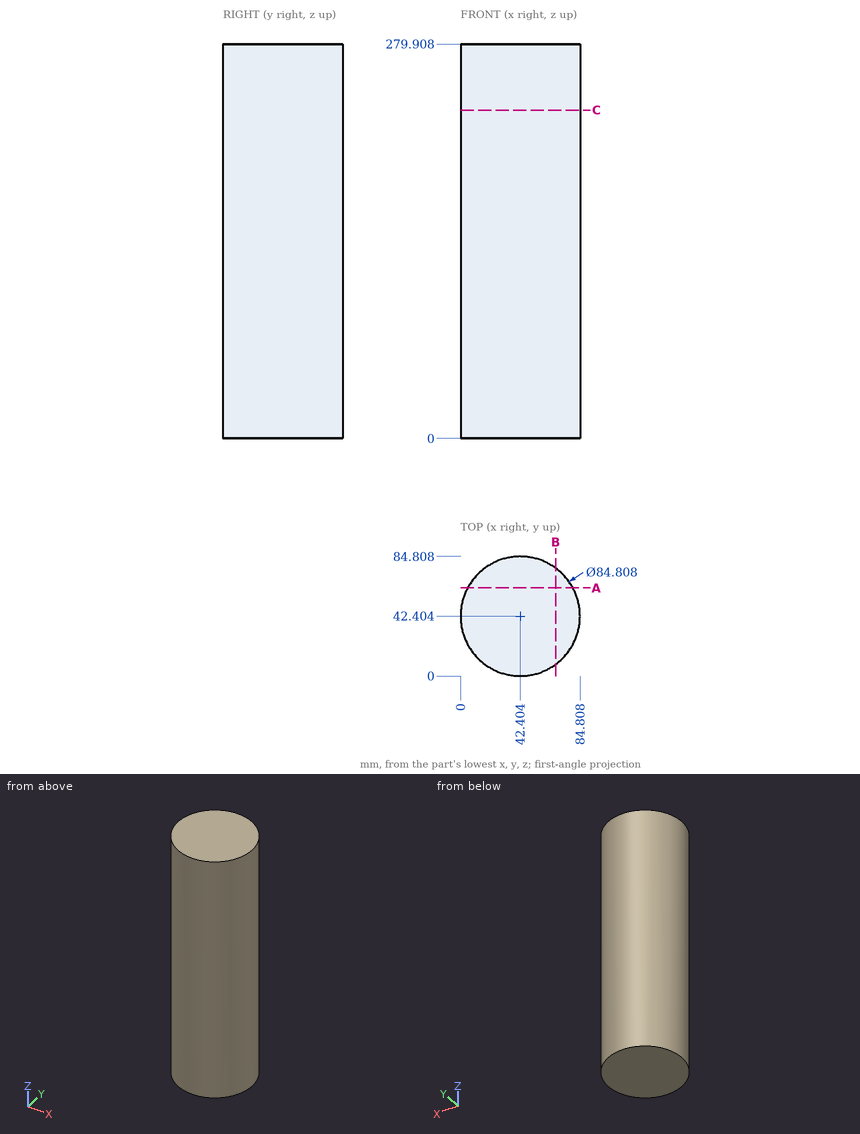
Can you work these out from the drawing? Everything is in mm from the part's minimum corner. Coordinates: 2 decimals unless noted, no trailing zeros. Order: outer loops, then holes, each group sorted by start corner. A loop starts at its lowest first (then second) coordinate and runs counter-clockwise, first axis right, second up. Notation, with made-up numbers: M 65,14 L 118,14 A27 cw 118,43 Z; hole C 85.5,78 d8. An arc over 180 degrees is marked long. Answer as CSV lines item,"result". Start each with the question number.
1. I want a section at B-B, the plane x = 67.5. Write out the boundary of the cut face in (y, z), and give its area (3 significant figures).
2. I need wall thicknesses on line 1 (X direction, y = 44, z = 201); line 2 (X direction, y = 57.5, z = 186); line 3 (Y direction, x = 31, z = 154). Which ranges of each line are inside material? Lowest first, please. Write a range as [from, to].
3. For pin 1 (6 mm diameter, centred on y = 20.5, z = 36, fed in from -X); pin 2 (12 mm diameter, centred on x = 17, z = 149.5, fed in from +Y); pin 3 (8 mm diameter, centred on y = 37, z = 31, fed in from +X), each with a flat end and sliding along its axis, tell me the tip position at first contact or that it passes through.
4. I want a section at A-A, the plane y = 62.5. Write out the boundary of the cut face in (x, z), and give its area (3 significant figures).
5. I want a section at C-C, the plane z = 233. Write out the boundary of the cut face in (x, y), and give its area (3 significant figures).
Recorded:
1,outline,"M 8.22,0 L 76.58,0 L 76.58,279.91 L 8.22,279.91 Z"
1,area,"19,100 mm2"
2,line 1,"x = [0.03, 84.78]"
2,line 2,"x = [2.78, 82.03]"
2,line 3,"y = [1.56, 83.25]"
3,pin 1,"stops at x = 4.45"
3,pin 2,"stops at y = 80.11"
3,pin 3,"stops at x = 84.78"
4,outline,"M 5.06,0 L 79.74,0 L 79.74,279.91 L 5.06,279.91 Z"
4,area,"20,900 mm2"
5,outline,"C 42.4,42.4 d84.81"
5,area,"5,650 mm2"
